```python
from build123d import *

# Parameters (mm, degrees)
SKETCH1_R           = 42.5
SKETCH1_R_2         = 20
BOSS_EXTRUDE1_DEPTH = 62.5
SKETCH2_R           = 17.5
BOSS_EXTRUDE2_DEPTH = 21.25
CIRPATTERN1_COUNT   = 2
CIRPATTERN1_ANGLE   = 300
SKETCH3_R           = 20
BOSS_EXTRUDE3_DEPTH = 12.5
BOSS_EXTRUDE4_DEPTH = 37.5
FILLET1_R           = 10


with BuildPart() as part:
    # Sketch1 → Boss-Extrude1 (new, symmetric)
    with BuildSketch(Plane.XY):
        Circle(SKETCH1_R)
        Circle(SKETCH1_R_2, mode=Mode.SUBTRACT)
    extrude(amount=BOSS_EXTRUDE1_DEPTH, both=True)

    # Sketch2 → Boss-Extrude2 (add, symmetric)
    with BuildSketch(Plane(origin=(0, 0, 0), x_dir=(1, 0, 0), z_dir=(0, 1, 0))):
        with BuildLine():
            Line((-20, -37.5), (-20, 37.5))
            Line((-20, 37.5), (-250, 37.5))
            ThreePointArc((-250, 37.5), (-287.5, 0), (-250, -37.5))
            Line((-250, -37.5), (-20, -37.5))
        make_face()
        with Locations(Location((-250, 0, 0), (0, 0, 270))):
            Circle(SKETCH2_R, mode=Mode.SUBTRACT)
    boss_extrude2 = extrude(amount=BOSS_EXTRUDE2_DEPTH, both=True)

    # CirPattern1: Boss-Extrude2 ×2 about axis
    cirpattern1_axis = Axis((0, 0, 62.5), (0, 0, 1))
    for i in range(1, CIRPATTERN1_COUNT):
        add(boss_extrude2.rotate(cirpattern1_axis, i * CIRPATTERN1_ANGLE / (CIRPATTERN1_COUNT - 1)))

    # Sketch3 → Boss-Extrude3 (add, symmetric)
    with BuildSketch(Plane.XY):
        with BuildLine():
            Line((0, -42.5), (-170, -42.5))
            Line((-170, -42.5), (-170, 97.5))
            Line((-170, 97.5), (-49.160292921, 168.194873881))
            Line((-49.160292921, 168.194873881), (36.683482506, 21.460943857))
            ThreePointArc((36.683482506, 21.460943857), (36.866923617, -21.144265015), (0, -42.5))
        make_face()
        Circle(SKETCH3_R, mode=Mode.SUBTRACT)
    extrude(amount=BOSS_EXTRUDE3_DEPTH, both=True)

    # Sketch4 → Boss-Extrude4 (add, symmetric)
    with BuildSketch(Plane.XY):
        Polygon((-49.160292921, 168.194873881), (-170, 97.5), (-170, -42.5), (-190, -42.5), (-190, 108.970588235), (-59.259560618, 185.457689178), align=None)
    extrude(amount=BOSS_EXTRUDE4_DEPTH, both=True)

    # Fillet1
    fillet1_edges = [part.edges().sort_by_distance(p)[0] for p in [
        (-36.806079661, -21.25, -25),
        (-36.806079661, 21.25, -25),
        (-66.659357171, 157.95739342, -25),
        (-66.659357171, 157.95739342, 25),
        (-103.343444163, 136.49609592, -25),
        (-170, 97.5, -25),
        (-103.343444163, 136.49609592, 25),
        (-170, 97.5, 25),
        (-170, 21.25, -25),
        (-170, 21.25, 25),
        (-170, -21.25, -25),
        (-170, -21.25, 25),
        (0, 42.5, -25),
        (-36.806079661, 21.25, 25),
        (0, 42.5, 25),
        (-36.806079661, -21.25, 25),
    ]]
    fillet(fillet1_edges, radius=FILLET1_R)


solid = part.part
```
Build history of the part. All positions in model axes, mm. A direction names the side the tool comes from. Give positions to 0.01 mm unless a question says otherwise; leave off trailing zeros. Loops run counter-clockwise (first coordinate to the right, second up) from the corner with the lowest first, then second, coordinate; pieces in that order, holes last. Notation, with made-up numbers: (4.5, 8) -> (53.5, 8) arc R27 ccw to (53.5, 34) -> close; hole circle Ø7 at (6, 8). An arc over 180 degrees is marked (long way). One line per question, with ' | ' between items. Start each with the question number.
1) Cut at B-B (z = -6). Give the cut face in (x, y).
2) Cut at D-D (z = -45). Give the cut face in (x, y), plus the area to 3 significant figures.
3) Pin check, flat tips, straight feed: pin 1 (4 mm diameter, centred on y = 133, z = -15, fed in from +X); pin 2 (12 mm diameter, centred on x = -33, z = 40.5, fed in from +Y); pin 3 (10 mm diameter, centred on y = 76.5, z = -34.5, fed in from +X); pin 4 (21 mm diameter, centred on x = -250, z = 0, fed in from -Y). Stop position of each tip, or through.
4) Cut at A-A (y = 0). Give the cut face in (x, z), plus the area to 3 significant figures.
5) Two-plate mould, pull along X, no slides. Class faces 5 (the flat face through (-170, -37, -25)), 6 (the flat face through (8.8, -18.3, -62.5)), 7 (the cylindrical face through (0.431, 43.834, -24.825)): released by +X, released by -X, zero draft, split by the parting line, or undercut.
6) Probe L1, parallel to X at y = -7, z = 0 (3 decimals); L2, parallel to Z at x = -66, y = 23; L3, parallel to Z at x = -110.5, y = 19. List the from-to ranges inside material, lowest first.
7) 3-axis set-ups, long thin cutter, end or side, ignore diameter. For faces 1 (the cylindrical face through (0.54, 43.76, 25.18)), 2 (the flat face through (-170, 62, -25)), 3 (the flat face through (-108, 21.25, 25)), 4 (the flat face through (-229, 21.25, -1)): which of +Z, -Z, +X, -X, +Y, -Y reach the whole face in a straight line?
8) Cut at C-C (z = -25.5). Count the separate pieces of the cut face and the enclosed holes in it, plus the area to 3 significant figures.
Return value:
1) outline: (-287.02, -21.25) -> (-266.44, -21.25) -> (-266.44, 21.25) -> (-287.02, 21.25) -> close; (-233.56, -21.25) -> (-190, -21.25) -> (-190, -42.5) -> (0, -42.5) arc R42.5 ccw to (36.68, 21.46) -> (-59.26, 185.46) -> (-76.66, 175.28) -> (-98.38, 212.89) -> (-135.18, 191.64) -> (-113.34, 153.82) -> (-190, 108.97) -> (-190, 21.25) -> (-233.56, 21.25) -> close; (-161.91, 237.94) -> (-151.62, 220.12) -> (-114.82, 241.37) -> (-125.11, 259.19) -> close; hole circle Ø40 at (0, 0)
2) outline: circle Ø85 at (0, 0); hole circle Ø40 at (0, 0) | area: 4,420 mm^2
3) pin 1: x = -51.1 | pin 2: y = 108.66 | pin 3: x = -16.74 | pin 4: through
4) outline: (-250, -37.5) -> (-42.5, -37.5) -> (-42.5, -62.5) -> (-20, -62.5) -> (-20, 62.5) -> (-42.5, 62.5) -> (-42.5, 37.5) -> (-250, 37.5) arc R37.5 ccw to start; (20, -62.5) -> (42.5, -62.5) -> (42.5, 62.5) -> (20, 62.5) -> close; hole circle Ø35 at (-250, 0) | area: 22,400 mm^2
5) face 5: undercut | face 6: zero draft | face 7: released by +X
6) L1: -287.5 to -267.5, -232.5 to -18.735, 18.735 to 41.92 | L2: -12.5 to 12.5 | L3: -37.5 to 37.5
7) face 1: +Z, +X, +Y | face 2: -Z | face 3: +Z | face 4: +Z, -Z, -X, +Y
8) separate pieces: 1 | enclosed holes: 2 | area: 28,800 mm^2
